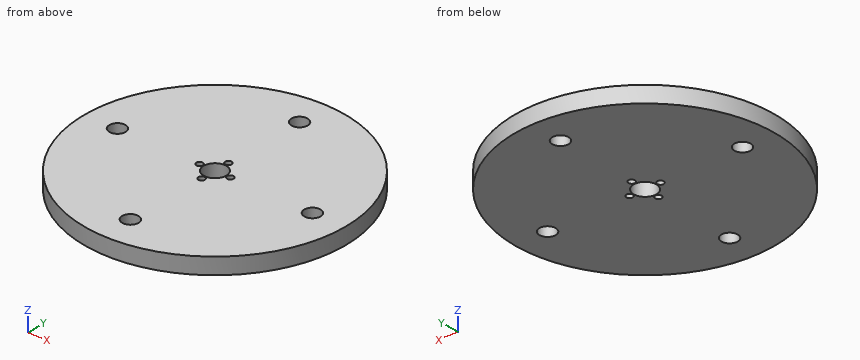
from build123d import *

# Parameters (mm, degrees)
F0_R     = 40
F0_R_2   = 2.5
F0_R_3   = 15
F0_R_4   = 1
F0_R_5   = 3.5
F1_DEPTH = 5


with BuildPart() as f1:
    # F0 (on Top) → F1 (new body)
    with BuildSketch(Plane.XY):
        Circle(F0_R)
        with Locations((0, -30)):
            Circle(F0_R_2, mode=Mode.SUBTRACT)
        with Locations((-30, 0)):
            Circle(F0_R_2, mode=Mode.SUBTRACT)
        Circle(F0_R_3, mode=Mode.SUBTRACT)
        with Locations((30, 0)):
            Circle(F0_R_2, mode=Mode.SUBTRACT)
        with Locations((0, 30)):
            Circle(F0_R_2, mode=Mode.SUBTRACT)
        Circle(F0_R_3)
        with Locations((0, -4.75)):
            Circle(F0_R_4, mode=Mode.SUBTRACT)
        with Locations((-4.75, 0)):
            Circle(F0_R_4, mode=Mode.SUBTRACT)
        Circle(F0_R_5, mode=Mode.SUBTRACT)
        with Locations((4.75, 0)):
            Circle(F0_R_4, mode=Mode.SUBTRACT)
        with Locations((0, 4.75)):
            Circle(F0_R_4, mode=Mode.SUBTRACT)
    extrude(amount=F1_DEPTH)


solid = f1.part
CAD build for the part. Positions are in the model's coordinates, mm. Round coordinates to 2 decimals unless told otherwise and drop trailing zeros. Write each loop counter-clockwise with the first axis right and the second up, starting at its lowest first coordinate (ties: lowest second). Pieces come first, ordered by that corner, then holes.
(1) Slice it at B-B, the plane z = 2. Count the separate pieces of the cut face and the enclosed holes in it, and give its area (3 significant figures).
(2) Drop flat-ended pins along their axis: P1, Ø3, axis at y = 3, z = 2.5, coming from the +X side; P2, Ø1.5, axis at x = -18.5, z = 4, coming from the -Y side; P3, Ø1.5, axis at y = -24, z = 3, coming from the +X side. Give the stop position or say it passes through.
(3) Probe line 1 along Y through (x, z) = (0, 3.75); line 2 along Y through (x, z) = (2, 1.3); line 3 along Y through (x, z) = (4.5, 3.1). List the from-to ranges inside material, lowest first.
(4) Slice it at D-D, the plane y = -31. Write the cut outline in (x, z), and give its area (3 significant figures).
(5) Slice it at A-A, the plane y = 0. Write the cut outline in (x, z), and give its area (3 significant figures).
From the geometry:
1. separate pieces: 1
1. enclosed holes: 9
1. area: 4,900 mm2
2. P1: stops at x = 39.97
2. P2: stops at y = -35.85
2. P3: stops at x = 32.55
3. line 1: y = -40 to -32.5, -27.5 to -5.75, -3.75 to -3.5, 3.5 to 3.75, 5.75 to 27.5, 32.5 to 40
3. line 2: y = -39.95 to -31.5, -28.5 to -2.87, 2.87 to 28.5, 31.5 to 39.95
3. line 3: y = -39.75 to -0.97, 0.97 to 39.75
4. outline: (-25.28, 0) - (-2.29, 0) - (-2.29, 5) - (-25.28, 5) - close; (2.29, 0) - (25.28, 0) - (25.28, 5) - (2.29, 5) - close
4. area: 230 mm2
5. outline: (-40, 0) - (-32.5, 0) - (-32.5, 5) - (-40, 5) - close; (-27.5, 0) - (-5.75, 0) - (-5.75, 5) - (-27.5, 5) - close; (-3.75, 0) - (-3.5, 0) - (-3.5, 5) - (-3.75, 5) - close; (3.5, 0) - (3.75, 0) - (3.75, 5) - (3.5, 5) - close; (5.75, 0) - (27.5, 0) - (27.5, 5) - (5.75, 5) - close; (32.5, 0) - (40, 0) - (40, 5) - (32.5, 5) - close
5. area: 295 mm2
